```python
from build123d import *

# Parameters (mm, degrees)
BOSS_EXTRUDE1_DEPTH                     = 40
SKETCH2_W                               = 40
SKETCH2_H                               = 40
BOSS_EXTRUDE2_DEPTH                     = 5
SKETCH3_W                               = 40
SKETCH3_H                               = 40
BOSS_EXTRUDE3_DEPTH                     = 10
CUT_EXTRUDE1_DEPTH                      = 30
CUT_EXTRUDE2_DEPTH                      = 30
CBORE_FOR_M5_HEX_HEAD_BOLT1_D           = 5.5
CBORE_FOR_M5_HEX_HEAD_BOLT1_DEPTH       = 5
CBORE_FOR_M5_HEX_HEAD_BOLT1_CBORE_D     = 12
CBORE_FOR_M5_HEX_HEAD_BOLT1_CBORE_DEPTH = 3
CHAMFER1_SIZE                           = 1


with BuildPart() as part:
    # Sketch1 → Boss-Extrude1 (new body)
    with BuildSketch(Plane(origin=(0, 20, 0), x_dir=(1, 0, 0), z_dir=(0, 1, 0))):
        Polygon((5, 4), (5, -20), (155.2, -20), (155.2, 4), (135.2, -16), (25, -16), align=None)
    extrude(amount=-BOSS_EXTRUDE1_DEPTH)

    # Sketch2 → Boss-Extrude2 (add)
    with BuildSketch(Plane.ZY.offset(-5)):
        Rectangle(SKETCH2_W, SKETCH2_H)
    extrude(amount=BOSS_EXTRUDE2_DEPTH)

    # Sketch3 → Boss-Extrude3 (add)
    with BuildSketch(Plane(origin=(155.2, 0, 0), x_dir=(0, 0, -1), z_dir=(1, 0, 0))):
        Rectangle(SKETCH3_W, SKETCH3_H)
    extrude(amount=BOSS_EXTRUDE3_DEPTH)

    # Sketch4 → Cut-Extrude1 (cut)
    with BuildSketch(Plane.XZ.offset(15)):
        Polygon((155.2, -4), (155.2, 16), (135.2, 16), align=None)
    extrude(amount=-CUT_EXTRUDE1_DEPTH, mode=Mode.SUBTRACT)

    # Sketch5 → Cut-Extrude2 (cut)
    with BuildSketch(Plane(origin=(0, 15, 0), x_dir=(1, 0, 0), z_dir=(0, 1, 0))):
        Polygon((5, 4), (5, -16), (25, -16), align=None)
    extrude(amount=-CUT_EXTRUDE2_DEPTH, mode=Mode.SUBTRACT)

    # Sketch6 → CBORE for M10 Hex Head Bolt1 (revolve, cut)
    with BuildSketch(Plane(origin=(0, -10, 10), x_dir=(0, 0, 1), z_dir=(0, 1, 0))):
        Polygon((0, 0), (0, 5), (6, 5), (6, 2), (2.75, 2), (2.75, 0), align=None)
    revolve(axis=Axis((-6.35, -10, 10), (1, 0, 0)), mode=Mode.SUBTRACT)

    # CBORE for M5 Hex Head Bolt1
    with Locations(Plane(origin=(5, 0, 0), x_dir=(0, 0, -1), z_dir=(1, 0, 0))):
        with Locations((10, 10)):
            CounterBoreHole(CBORE_FOR_M5_HEX_HEAD_BOLT1_D / 2, CBORE_FOR_M5_HEX_HEAD_BOLT1_CBORE_D / 2, CBORE_FOR_M5_HEX_HEAD_BOLT1_CBORE_DEPTH, depth=CBORE_FOR_M5_HEX_HEAD_BOLT1_DEPTH)

    # Chamfer1
    chamfer1_edges = [part.edges().sort_by_distance(p)[0] for p in [
        (82.6, -20, 20),
        (5, 20, -12),
        (5, 0, -20),
        (2.5, 20, -20),
        (5, -20, -12),
        (145.2, -20, 6),
        (2.5, -20, -20),
        (0, 20, 0),
        (0, -20, 0),
        (0, 0, 20),
        (80.1, -20, 16),
        (155.2, 20, -12),
        (160.2, 20, -20),
        (155.2, -20, -12),
        (155.2, 0, -20),
        (160.2, -20, -20),
        (165.2, 20, 0),
        (165.2, 0, 20),
        (165.2, -20, 0),
        (165.2, 0, -20),
        (145.2, 15, 6),
        (145.2, -15, 6),
        (15, -20, 6),
        (15, -15, 6),
        (15, 15, 6),
        (80.1, 20, 16),
        (145.2, 20, 6),
        (82.6, 20, 20),
        (15, 20, 6),
    ]]
    chamfer(chamfer1_edges, length=CHAMFER1_SIZE)


solid = part.part
```
Can you work these out from the model? Positions are in its coordinate system, mm. A direction names the side the tool comes from. Coordinates: 2 decimals unless noted, no trailing zeros. Loops run counter-clockwise (first coordinate to the right, second up) from the corner with the lowest first, then second, coordinate; pieces in that order, holes last. Notation, with made-up numbers: (11.5, 21) -> (59.5, 21) arc R10 cw to (59.5, 26) -> close; hole circle Ø7 at (24, 42.5). An arc over 180 degrees is marked (long way). Put each result on its own line as item: value. Start each with the question number.
Q1. If I drill on line 1 (Y direction, x = 3, z = 10); line 2 (X direction, y = -5, z = -7); line 3 (X direction, y = -12, z = 8), over which ranges is the centre line in solid material (lowest first)? Write a range as [from, to].
Q2. I want a section at D-D (y = 2.5). Write out the boundary of the cut face in (x, z), plus the area to 3 significant figures.
Q3. I want a section at B-B (z = -10). Write out the boundary of the cut face in (x, y).
Q4. I want a section at A-A (y = 10). Write out the boundary of the cut face in (x, z), plus the area to 3 significant figures.
Q5. Thinking about a two-plate mould opening in Y: for faces 4 (the face through (15, 18, 6)), 5 (the face through (145.42, 15.49, 6.5)), 6 (the face through (88, 20, 18)), which applies, pulls with the +Y half, pulls with the -Y half, needs draft (parallel to the pull), parting line crosses it, or undercut?
Q6. I want a section at C-C (x = 51). Write out the boundary of the cut face in (y, z).
Q7. For faces 1 (the face through (155.2, 0, -1)), 2 (the face through (145.69, -19.49, 6.2)), 3 (the face through (0.99, 12.32, -8.52)), which set-ups out of +Z, -Z, +X, -X, +Y, -Y let a thin tool reach every point of the face, with its end or its side?
Q8. I'm going to push flat-ended pins straight in: P1, Ø5, axis at x = 23.5, y = -14, coming from the -Z side; P2, Ø1.5, axis at x = 27, y = -1.5, coming from the -Z side. Where does each tip first touch, or does it pass through?
Taken from the geometry:
1. line 1: y = [-20, -16], [-4, 20]
1. line 2: x = [0, 5], [155.2, 165.2]
1. line 3: x = [0, 2], [155.2, 165.2]
2. outline: (0, -20) -> (4, -20) -> (5, -19) -> (5, 16) -> (155.2, 16) -> (155.2, -19) -> (156.2, -20) -> (164.2, -20) -> (165.2, -19) -> (165.2, 19) -> (164.2, 20) -> (1, 20) -> (0, 19) -> close
2. area: 1,200 mm2
3. outline: (0, -19) -> (1, -20) -> (4, -20) -> (5, -19) -> (5, 4) -> (2, 4) -> (2, 7.25) -> (0, 7.25) -> close; (0, 12.75) -> (2, 12.75) -> (2, 16) -> (5, 16) -> (5, 19) -> (4, 20) -> (1, 20) -> (0, 19) -> close; (155.2, -19) -> (156.2, -20) -> (164.2, -20) -> (165.2, -19) -> (165.2, 19) -> (164.2, 20) -> (156.2, 20) -> (155.2, 19) -> close
4. outline: (0, -20) -> (4, -20) -> (5, -19) -> (5, -16) -> (2, -16) -> (2, -12.75) -> (0, -12.75) -> close; (0, -7.25) -> (2, -7.25) -> (2, -4) -> (5, -4) -> (5, 16) -> (155.2, 16) -> (155.2, -19) -> (156.2, -20) -> (164.2, -20) -> (165.2, -19) -> (165.2, 19) -> (164.2, 20) -> (1, 20) -> (0, 19) -> close
4. area: 1,150 mm2
5. face 4: needs draft
5. face 5: undercut
5. face 6: pulls with the +Y half
6. outline: (-20, 17) -> (-19, 16) -> (19, 16) -> (20, 17) -> (20, 19) -> (19, 20) -> (-19, 20) -> (-20, 19) -> close
7. face 1: -Z
7. face 2: -Z, -Y
7. face 3: -X
8. P1: stops at z = 13
8. P2: stops at z = 16
